Geometry: final body of the model. Coordinates: model frame, mm. Face numbers are marked on the shaded views. Round coordinates to 2 decimals unless told otherwise and drop trailing zeros. Loops run counter-clockwise (first coordinate to the right, second up) from the corner with the lowest first, then second, coordinate; pieces in that order, holes last. Notation, with made-up numbers: M 76,64.25 L 103,64.25 A21 ccw 103,90.25 Z; hole C 84,39.5 d9. An arc over 180 degrees is marked long. Write each question's results on one line, items separated by ' | '.
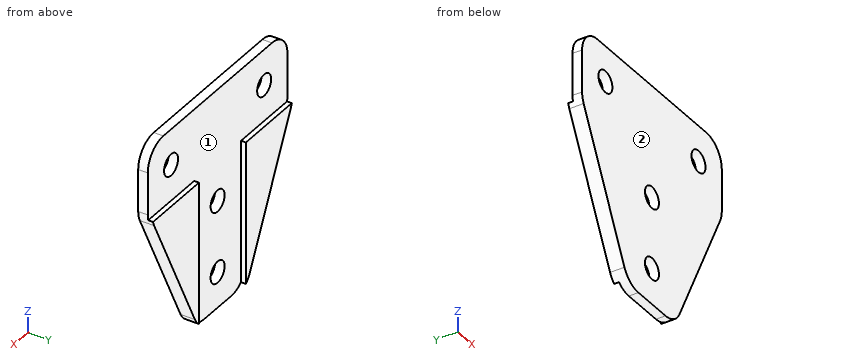
```python
from build123d import *

# Parameters (mm, degrees)
EXTRUDE_1_DEPTH     = 3
SKETCH_2_R          = 2.25
CUT_EXTRUDE_1_DEPTH = 3
FILLET_1_R          = 5
CUT_EXTRUDE_2_DEPTH = 1


with BuildPart() as part:
    # ｽｹｯﾁ1 → ﾎﾞｽ - 押し出し1 (new body)
    with BuildSketch(Plane(origin=(0, 0, 0), x_dir=(1, 0, 0), z_dir=(0, 1, 0))):
        Polygon((0, 0), (45, 0), (45, 15), (30, 46), (15, 46), (0, 15), align=None)
    extrude(amount=EXTRUDE_1_DEPTH)

    # ｽｹｯﾁ2 → ｶｯﾄ - 押し出し1 (cut)
    with BuildSketch(Plane(origin=(0, 3, 0), x_dir=(1, 0, 0), z_dir=(0, 1, 0))):
        with Locations((7.5, 7.5)):
            Circle(SKETCH_2_R)
        with Locations((22.5, 38.5)):
            Circle(SKETCH_2_R)
        with Locations((22.5, 23.5)):
            Circle(SKETCH_2_R)
        with Locations((37.5, 7.5)):
            Circle(SKETCH_2_R)
    extrude(amount=-CUT_EXTRUDE_1_DEPTH, mode=Mode.SUBTRACT)

    # ﾌｨﾚｯﾄ1
    fillet_1_edges = [part.edges().sort_by_distance(p)[0] for p in [
        (0, 1.5, -15),
        (15, 1.5, -46),
        (30, 1.5, -46),
        (45, 1.5, -15),
        (45, 1.5, 0),
        (0, 1.5, 0),
    ]]
    fillet(fillet_1_edges, radius=FILLET_1_R)

    # ｽｹｯﾁ3 → ｶｯﾄ - 押し出し2 (cut)
    with BuildSketch(Plane(origin=(0, 3, 0), x_dir=(1, 0, 0), z_dir=(0, 1, 0))):
        Polygon((14.95, 46), (30.05, 46), (30.05, 15.05), (45, 15.05), (45, 0), (0, 0), (0, 15.05), (14.95, 15.05), align=None)
    extrude(amount=-CUT_EXTRUDE_2_DEPTH, mode=Mode.SUBTRACT)


solid = part.part
```
1. Ray query, probe 1 along Z at (x, y) = (22.5, 0.9); probe 2 along X at (y, z) = (1.3, -7.5); probe 3 along X at (y, z) = (1, -37). Return the intervals inside material, ascending.
Answer key:
probe 1: z = -46 to -40.75, -36.25 to -25.75, -21.25 to 0 | probe 2: x = 0 to 5.25, 9.75 to 35.25, 39.75 to 45 | probe 3: x = 10.65 to 20.82, 24.18 to 34.35
2. Section C-C (z = -7.5). Output: boundary loops of the cut face in (x, y).
Answer key:
outline: M 0,0 L 5.25,0 L 5.25,2 L 0,2 Z; M 9.75,0 L 35.25,0 L 35.25,2 L 9.75,2 Z; M 39.75,0 L 45,0 L 45,2 L 39.75,2 Z
3. Section A-A (y = 1.3). Output: boundary loops of the cut face in (x, z), then the cut area to 3 significant figures.
Answer key:
outline: M 0,-13.85 A5 ccw 0.5,-16.03 L 13.63,-43.18 A5 ccw 18.14,-46 L 26.86,-46 A5 ccw 31.37,-43.18 L 44.5,-16.03 A5 ccw 45,-13.85 L 45,-5 A5 ccw 40,0 L 5,0 A5 ccw 0,-5 Z; hole C 7.5,-7.5 d4.5; hole C 22.5,-38.5 d4.5; hole C 22.5,-23.5 d4.5; hole C 37.5,-7.5 d4.5 | area: 1,530 mm²
4. Pin query (flat end, axial travel): P1, Ø0.5, axis at y = 2.5, z = -29, coming from the -X side; P2, Ø10, axis at x = 26, z = -28, coming from the +Y side; P3, Ø0.8, axis at x = 34, y = 2.5, coming from the +Z side; P4, Ø8, axis at x = 21, z = -38.5, coming from the +Y side. Return the tip coordinate at first contact, or that it passes through.
Answer key:
P1: stops at x = 6.65 | P2: stops at y = 3 | P3: stops at z = -15.05 | P4: stops at y = 2
5. Section D-D (x = 22.5). Output: boundary loops of the cut face in (y, z), then the cut area to 3 significant figures.
Answer key:
outline: M 0,-46 L 2,-46 L 2,-40.75 L 0,-40.75 Z; M 0,-36.25 L 2,-36.25 L 2,-25.75 L 0,-25.75 Z; M 0,-21.25 L 2,-21.25 L 2,0 L 0,0 Z | area: 74.0 mm²
6. Draft query along X for the marked faces 1 and 2. Return one class per face: pulls with the +X half, pulls with the -X half, needs draft (parallel to the pull), parting line crosses it, or undercut.
Answer key:
face 1: undercut | face 2: needs draft
7. Section B-B (x = 37.5). Output: boundary loops of the cut face in (y, z).
Answer key:
outline: M 0,-30.5 L 3,-30.5 L 3,-15.05 L 2,-15.05 L 2,-9.75 L 0,-9.75 Z; M 0,-5.25 L 2,-5.25 L 2,0 L 0,0 Z
